```python
from build123d import *

# Parameters (mm, degrees)
SKETCH1_W            = 35
SKETCH1_H            = 6
BOSS_EXTRUDE1_DEPTH  = 12
BOSS_EXTRUDE2_DEPTH  = 12
SKETCH4_W            = 6
SKETCH4_H            = 13.146428929
CUT_EXTRUDE1_DEPTH   = 8
CUT_EXTRUDE2_DEPTH   = 8
LPATTERN2_COUNT      = 10
LPATTERN2_PITCH      = 2
MIRROR1_COPY_1_DEPTH = 8
MIRROR1_COPY_2_DEPTH = 8
MIRROR1_COPY_3_DEPTH = 8
MIRROR1_COPY_4_DEPTH = 8
MIRROR1_COPY_5_DEPTH = 8
MIRROR1_COPY_6_DEPTH = 8
MIRROR1_COPY_7_DEPTH = 8
MIRROR1_COPY_8_DEPTH = 8
MIRROR1_COPY_9_DEPTH = 8
CUT_EXTRUDE3_DEPTH   = 25.961542292
BOSS_EXTRUDE3_DEPTH  = 1
BOSS_EXTRUDE4_DEPTH  = 1


with BuildPart() as part:
    # Sketch1 → Boss-Extrude1 (new body)
    with BuildSketch(Plane.XY):
        Rectangle(SKETCH1_W, SKETCH1_H)
    extrude(amount=BOSS_EXTRUDE1_DEPTH)

    # Sketch2 → Boss-Extrude2 (add)
    with BuildSketch(Plane.XY.offset(12)):
        with BuildLine():
            Line((-17.5, -3), (17.5, -3))
            ThreePointArc((17.5, -3), (0, -10.146428929), (-17.5, -3))
        make_face()
    extrude(amount=-BOSS_EXTRUDE2_DEPTH)

    # Sketch4 → Cut-Extrude1 (cut)
    with BuildSketch(Plane.XY.offset(12)):
        with Locations((0, -3.573214465)):
            Rectangle(SKETCH4_W, SKETCH4_H)
    extrude(amount=-CUT_EXTRUDE1_DEPTH, mode=Mode.SUBTRACT)

    # Sketch5 → Cut-Extrude2 (cut)
    with BuildSketch(Plane.XY.offset(12)):
        with BuildLine():
            Line((3, 2), (3, 4))
            ThreePointArc((3, 4), (3.084360941, 3.705850588), (3.311797753, 3.501123596))
            ThreePointArc((3.311797753, 3.501123596), (3.461937846, 3.442388286), (3.619565217, 3.408543109))
            ThreePointArc((3.619565217, 3.408543109), (3.712771412, 3.358731646), (3.75, 3.259824575))
            Line((3.75, 3.259824575), (3.75, 2.740175425))
            ThreePointArc((3.75, 2.740175425), (3.712771412, 2.641268354), (3.619565217, 2.591456891))
            ThreePointArc((3.619565217, 2.591456891), (3.461937846, 2.557611714), (3.311797753, 2.498876404))
            ThreePointArc((3.311797753, 2.498876404), (3.084360941, 2.294149412), (3, 2))
        make_face()
    cut_extrude2 = extrude(amount=-CUT_EXTRUDE2_DEPTH, mode=Mode.SUBTRACT)

    # LPattern2: Cut-Extrude2 ×10
    with Locations(*[(0, -i * LPATTERN2_PITCH, 0) for i in range(1, LPATTERN2_COUNT)]):
        add(cut_extrude2, mode=Mode.SUBTRACT)

    # Mirror1: Cut-Extrude2 across plane
    add(cut_extrude2.mirror(Plane(origin=(0, 0, 0), x_dir=(0, 0, 1), z_dir=(1, 0, 0))), mode=Mode.SUBTRACT)

    # Mirror1 copy 1 sketch → Mirror1 copy 1 (cut)
    with BuildSketch(Plane(origin=(0, -2, 12), x_dir=(-1, 0, 0), z_dir=(0, 0, 1))):
        with BuildLine():
            Line((3, -2), (3, -4))
            ThreePointArc((3, -4), (3.084360941, -3.705850588), (3.311797753, -3.501123596))
            ThreePointArc((3.311797753, -3.501123596), (3.461937846, -3.442388286), (3.619565217, -3.408543109))
            ThreePointArc((3.619565217, -3.408543109), (3.712771412, -3.358731646), (3.75, -3.259824575))
            Line((3.75, -3.259824575), (3.75, -2.740175425))
            ThreePointArc((3.75, -2.740175425), (3.712771412, -2.641268354), (3.619565217, -2.591456891))
            ThreePointArc((3.619565217, -2.591456891), (3.461937846, -2.557611714), (3.311797753, -2.498876404))
            ThreePointArc((3.311797753, -2.498876404), (3.084360941, -2.294149412), (3, -2))
        make_face()
    extrude(amount=-MIRROR1_COPY_1_DEPTH, mode=Mode.SUBTRACT)

    # Mirror1 copy 2 sketch → Mirror1 copy 2 (cut)
    with BuildSketch(Plane(origin=(0, -4, 12), x_dir=(-1, 0, 0), z_dir=(0, 0, 1))):
        with BuildLine():
            Line((3, -2), (3, -4))
            ThreePointArc((3, -4), (3.084360941, -3.705850588), (3.311797753, -3.501123596))
            ThreePointArc((3.311797753, -3.501123596), (3.461937846, -3.442388286), (3.619565217, -3.408543109))
            ThreePointArc((3.619565217, -3.408543109), (3.712771412, -3.358731646), (3.75, -3.259824575))
            Line((3.75, -3.259824575), (3.75, -2.740175425))
            ThreePointArc((3.75, -2.740175425), (3.712771412, -2.641268354), (3.619565217, -2.591456891))
            ThreePointArc((3.619565217, -2.591456891), (3.461937846, -2.557611714), (3.311797753, -2.498876404))
            ThreePointArc((3.311797753, -2.498876404), (3.084360941, -2.294149412), (3, -2))
        make_face()
    extrude(amount=-MIRROR1_COPY_2_DEPTH, mode=Mode.SUBTRACT)

    # Mirror1 copy 3 sketch → Mirror1 copy 3 (cut)
    with BuildSketch(Plane(origin=(0, -6, 12), x_dir=(-1, 0, 0), z_dir=(0, 0, 1))):
        with BuildLine():
            Line((3, -2), (3, -4))
            ThreePointArc((3, -4), (3.084360941, -3.705850588), (3.311797753, -3.501123596))
            ThreePointArc((3.311797753, -3.501123596), (3.461937846, -3.442388286), (3.619565217, -3.408543109))
            ThreePointArc((3.619565217, -3.408543109), (3.712771412, -3.358731646), (3.75, -3.259824575))
            Line((3.75, -3.259824575), (3.75, -2.740175425))
            ThreePointArc((3.75, -2.740175425), (3.712771412, -2.641268354), (3.619565217, -2.591456891))
            ThreePointArc((3.619565217, -2.591456891), (3.461937846, -2.557611714), (3.311797753, -2.498876404))
            ThreePointArc((3.311797753, -2.498876404), (3.084360941, -2.294149412), (3, -2))
        make_face()
    extrude(amount=-MIRROR1_COPY_3_DEPTH, mode=Mode.SUBTRACT)

    # Mirror1 copy 4 sketch → Mirror1 copy 4 (cut)
    with BuildSketch(Plane(origin=(0, -8, 12), x_dir=(-1, 0, 0), z_dir=(0, 0, 1))):
        with BuildLine():
            Line((3, -2), (3, -4))
            ThreePointArc((3, -4), (3.084360941, -3.705850588), (3.311797753, -3.501123596))
            ThreePointArc((3.311797753, -3.501123596), (3.461937846, -3.442388286), (3.619565217, -3.408543109))
            ThreePointArc((3.619565217, -3.408543109), (3.712771412, -3.358731646), (3.75, -3.259824575))
            Line((3.75, -3.259824575), (3.75, -2.740175425))
            ThreePointArc((3.75, -2.740175425), (3.712771412, -2.641268354), (3.619565217, -2.591456891))
            ThreePointArc((3.619565217, -2.591456891), (3.461937846, -2.557611714), (3.311797753, -2.498876404))
            ThreePointArc((3.311797753, -2.498876404), (3.084360941, -2.294149412), (3, -2))
        make_face()
    extrude(amount=-MIRROR1_COPY_4_DEPTH, mode=Mode.SUBTRACT)

    # Mirror1 copy 5 sketch → Mirror1 copy 5 (cut)
    with BuildSketch(Plane(origin=(0, -10, 12), x_dir=(-1, 0, 0), z_dir=(0, 0, 1))):
        with BuildLine():
            Line((3, -2), (3, -4))
            ThreePointArc((3, -4), (3.084360941, -3.705850588), (3.311797753, -3.501123596))
            ThreePointArc((3.311797753, -3.501123596), (3.461937846, -3.442388286), (3.619565217, -3.408543109))
            ThreePointArc((3.619565217, -3.408543109), (3.712771412, -3.358731646), (3.75, -3.259824575))
            Line((3.75, -3.259824575), (3.75, -2.740175425))
            ThreePointArc((3.75, -2.740175425), (3.712771412, -2.641268354), (3.619565217, -2.591456891))
            ThreePointArc((3.619565217, -2.591456891), (3.461937846, -2.557611714), (3.311797753, -2.498876404))
            ThreePointArc((3.311797753, -2.498876404), (3.084360941, -2.294149412), (3, -2))
        make_face()
    extrude(amount=-MIRROR1_COPY_5_DEPTH, mode=Mode.SUBTRACT)

    # Mirror1 copy 6 sketch → Mirror1 copy 6 (cut)
    with BuildSketch(Plane(origin=(0, -12, 12), x_dir=(-1, 0, 0), z_dir=(0, 0, 1))):
        with BuildLine():
            Line((3, -2), (3, -4))
            ThreePointArc((3, -4), (3.084360941, -3.705850588), (3.311797753, -3.501123596))
            ThreePointArc((3.311797753, -3.501123596), (3.461937846, -3.442388286), (3.619565217, -3.408543109))
            ThreePointArc((3.619565217, -3.408543109), (3.712771412, -3.358731646), (3.75, -3.259824575))
            Line((3.75, -3.259824575), (3.75, -2.740175425))
            ThreePointArc((3.75, -2.740175425), (3.712771412, -2.641268354), (3.619565217, -2.591456891))
            ThreePointArc((3.619565217, -2.591456891), (3.461937846, -2.557611714), (3.311797753, -2.498876404))
            ThreePointArc((3.311797753, -2.498876404), (3.084360941, -2.294149412), (3, -2))
        make_face()
    extrude(amount=-MIRROR1_COPY_6_DEPTH, mode=Mode.SUBTRACT)

    # Mirror1 copy 7 sketch → Mirror1 copy 7 (cut)
    with BuildSketch(Plane(origin=(0, -14, 12), x_dir=(-1, 0, 0), z_dir=(0, 0, 1))):
        with BuildLine():
            Line((3, -2), (3, -4))
            ThreePointArc((3, -4), (3.084360941, -3.705850588), (3.311797753, -3.501123596))
            ThreePointArc((3.311797753, -3.501123596), (3.461937846, -3.442388286), (3.619565217, -3.408543109))
            ThreePointArc((3.619565217, -3.408543109), (3.712771412, -3.358731646), (3.75, -3.259824575))
            Line((3.75, -3.259824575), (3.75, -2.740175425))
            ThreePointArc((3.75, -2.740175425), (3.712771412, -2.641268354), (3.619565217, -2.591456891))
            ThreePointArc((3.619565217, -2.591456891), (3.461937846, -2.557611714), (3.311797753, -2.498876404))
            ThreePointArc((3.311797753, -2.498876404), (3.084360941, -2.294149412), (3, -2))
        make_face()
    extrude(amount=-MIRROR1_COPY_7_DEPTH, mode=Mode.SUBTRACT)

    # Mirror1 copy 8 sketch → Mirror1 copy 8 (cut)
    with BuildSketch(Plane(origin=(0, -16, 12), x_dir=(-1, 0, 0), z_dir=(0, 0, 1))):
        with BuildLine():
            Line((3, -2), (3, -4))
            ThreePointArc((3, -4), (3.084360941, -3.705850588), (3.311797753, -3.501123596))
            ThreePointArc((3.311797753, -3.501123596), (3.461937846, -3.442388286), (3.619565217, -3.408543109))
            ThreePointArc((3.619565217, -3.408543109), (3.712771412, -3.358731646), (3.75, -3.259824575))
            Line((3.75, -3.259824575), (3.75, -2.740175425))
            ThreePointArc((3.75, -2.740175425), (3.712771412, -2.641268354), (3.619565217, -2.591456891))
            ThreePointArc((3.619565217, -2.591456891), (3.461937846, -2.557611714), (3.311797753, -2.498876404))
            ThreePointArc((3.311797753, -2.498876404), (3.084360941, -2.294149412), (3, -2))
        make_face()
    extrude(amount=-MIRROR1_COPY_8_DEPTH, mode=Mode.SUBTRACT)

    # Mirror1 copy 9 sketch → Mirror1 copy 9 (cut)
    with BuildSketch(Plane(origin=(0, -18, 12), x_dir=(-1, 0, 0), z_dir=(0, 0, 1))):
        with BuildLine():
            Line((3, -2), (3, -4))
            ThreePointArc((3, -4), (3.084360941, -3.705850588), (3.311797753, -3.501123596))
            ThreePointArc((3.311797753, -3.501123596), (3.461937846, -3.442388286), (3.619565217, -3.408543109))
            ThreePointArc((3.619565217, -3.408543109), (3.712771412, -3.358731646), (3.75, -3.259824575))
            Line((3.75, -3.259824575), (3.75, -2.740175425))
            ThreePointArc((3.75, -2.740175425), (3.712771412, -2.641268354), (3.619565217, -2.591456891))
            ThreePointArc((3.619565217, -2.591456891), (3.461937846, -2.557611714), (3.311797753, -2.498876404))
            ThreePointArc((3.311797753, -2.498876404), (3.084360941, -2.294149412), (3, -2))
        make_face()
    extrude(amount=-MIRROR1_COPY_9_DEPTH, mode=Mode.SUBTRACT)

    # Sketch6 → Cut-Extrude3 (cut, through all)
    with BuildSketch(Plane(origin=(0, 3, 0), x_dir=(1, 0, 0), z_dir=(0, 1, 0))):
        Polygon((7.187822174, -12), (-7.187822174, -12), (-13.25, -1.5), (13.25, -1.5), align=None)
    extrude(amount=-CUT_EXTRUDE3_DEPTH, mode=Mode.SUBTRACT)

    # Sketch7 → Boss-Extrude3 (add)
    with BuildSketch(Plane.XY.offset(12)):
        with BuildLine():
            Line((17.5, 3), (7.187822174, 3))
            Line((7.187822174, 3), (7.187822174, -10.133129639))
            ThreePointArc((7.187822174, -10.133129639), (12.675182552, -7.847524657), (17.5, -4.375313452))
            Line((17.5, -4.375313452), (17.5, 3))
        make_face()
    boss_extrude3 = extrude(amount=BOSS_EXTRUDE3_DEPTH)

    # Mirror2: Boss-Extrude3 across plane
    add(boss_extrude3.mirror(Plane(origin=(0, 0, 0), x_dir=(0, 0, 1), z_dir=(1, 0, 0))))

    # Sketch8 → Boss-Extrude4 (add)
    with BuildSketch(Plane(origin=(0, 0, 0), x_dir=(-1, 0, 0), z_dir=(0, 0, -1))):
        with BuildLine():
            Line((17.5, -4.375313452), (17.5, -3))
            ThreePointArc((17.5, -3), (0, -10.146428929), (-17.5, -3))
            Line((-17.5, -3), (-17.5, -4.375313452))
            ThreePointArc((-17.5, -4.375313452), (0, -11.146428929), (17.5, -4.375313452))
        make_face()
    extrude(amount=-BOSS_EXTRUDE4_DEPTH)


solid = part.part
```
Could you check a few things on this model? Use its own coordinates, in mm. A direction names the side the tool comes from. Round coordinates to 2 decimals unless told otherwise and drop trailing zeros. Loops run counter-clockwise (first coordinate to the right, second up) from the corner with the lowest first, then second, coordinate; pieces in that order, holes last. Notation, with made-up numbers: (63.25, -11) -> (88.25, -11) arc R31 ccw to (88.25, 14) -> close; hole circle Ø1 at (-1.75, 24.5). An arc over 180 degrees is marked (long way). One line per question, with ' | ' between items.
(1) For faces 1 (the face through (-12.3, -7.1, 12)), 2 (the face through (8.701, -8.583, 10.244)), 3 (the face through (7.188, -3.5, 12.5)), which set-ups out of +Z, -Z, +X, -X, +Y, -Y let a thin tool reach every point of the face, with its end or its side?
Model answer:
face 1: -X, -Y | face 2: -Y | face 3: +Z, +Y, -Y
(2) Thinking about a two-plate mould opening in Z: for faces 4 (the face through (0, -2, 0)), 5 (the face through (12.3, -7.1, 12)), 6 (the face through (-17.5, 0, 6)), 7 (the face through (0.1, -10.4, 1)), which applies, released by +Z, released by -Z, zero draft, split by the parting line, or undercut?
Model answer:
face 4: released by -Z | face 5: undercut | face 6: zero draft | face 7: undercut
(3) If we section it at C-C on y = -7.25: List the corners of the cut face in (x, z) for me, and give its area (3 significant figures).
Model answer:
outline: (-13.69, 0) -> (13.69, 0) -> (13.69, 1) -> (11.68, 1) -> (11.68, 1.5) -> (-11.68, 1.5) -> (-11.68, 1) -> (-13.69, 1) -> close; (-13.69, 12) -> (-11.68, 12) -> (-11.68, 4.22) -> (-7.19, 12) -> (-7.19, 13) -> (-13.69, 13) -> close; (7.19, 12) -> (11.68, 4.22) -> (11.68, 12) -> (13.69, 12) -> (13.69, 13) -> (7.19, 13) -> close | area: 87.0 mm^2
(4) If we section it at D-D on y = -0.5: List the corners of the cut face in (x, z) for me, and give its area (3 significant figures).
Model answer:
outline: (-17.5, 0) -> (17.5, 0) -> (17.5, 13) -> (7.19, 13) -> (7.19, 12) -> (13.25, 1.5) -> (-13.25, 1.5) -> (-7.19, 12) -> (-7.19, 13) -> (-17.5, 13) -> close | area: 226 mm^2
(5) If we section it at B-B on x = -10: List the corners of the cut face in (y, z) for me, and give its area (3 significant figures).
Model answer:
outline: (-9.15, 0) -> (3, 0) -> (3, 1.5) -> (-8.06, 1.5) -> (-8.06, 1) -> (-9.15, 1) -> close; (-9.15, 12) -> (-8.06, 12) -> (-8.06, 7.13) -> (3, 7.13) -> (3, 13) -> (-9.15, 13) -> close | area: 83.7 mm^2
(6) If we section it at A-A on z = 5.5: List the corners of the cut face in (x, y) for me, and give its area (3 significant figures).
Model answer:
outline: (-17.5, -3) arc R25 ccw to (-10.94, -7.63) -> (-10.94, 3) -> (-17.5, 3) -> close; (10.94, -7.63) arc R25 ccw to (17.5, -3) -> (17.5, 3) -> (10.94, 3) -> close | area: 113 mm^2
(7) If I drill on probe 1 along Z at (x, y) = (-13, -7.5); probe 2 along Z at (x, y) = (3, 1.5); probe 3 along Z at (x, y) = (7, -9.75), over which ranges is the centre line in solid material (lowest first)?
Model answer:
probe 1: z = 0 to 1, 12 to 13 | probe 2: z = 0 to 1.5 | probe 3: z = 0 to 1
(8) For pin 1 Ø1.1 at (y, z) = (-6.5, 12.5) entering from +X; pin 2 Ø3 at (y, z) = (-9.5, 9) entering from +X, each with a flat end and sliding along its axis, tell me the tip position at first contact or that it passes through.
Model answer:
pin 1: stops at x = 15.6 | pin 2: stops at x = 10.13
